Build history of the part. All positions in model axes, mm. Round coordinates to 2 decimals unless told otherwise and drop trailing zeros. Write each loop counter-clockwise with the first axis right and the second up, starting at its lowest first coordinate (ties: lowest second). Pieces come first, ordered by that corner, then holes. Notation, with made-up numbers: (76.5, -25.75) -> (132.5, -25.75) arc R22 cw to (132.5, -12.75) -> close; hole circle Ø1 at (77.25, 55). An arc over 180 degrees is marked (long way). Answer in a Markdown table with one row per item.
```python
from build123d import *

# Parameters (mm, degrees)
SZKIC2_R                         = 5
DODANIE_WYCI_GNI_CIE1_DEPTH      = 175
DODANIE_WYCI_GNI_CIE2_DEPTH      = 15
DODANIE_WYCI_GNI_CIE2_DEPTH_BACK = 15
SZKIC3_R                         = 1
ZAOKR_GLENIE1_R                  = 5


with BuildPart() as part:
    # Szkic2 → Dodanie-wyci_gni_cie1 (new body)
    with BuildSketch(Plane(origin=(0, 0, 0), x_dir=(1, 0, 0), z_dir=(0, 1, 0))):
        with Locations(Location((0, 0, 0), (0, 0, 270))):
            Circle(SZKIC2_R)
    extrude(amount=DODANIE_WYCI_GNI_CIE1_DEPTH)

    # Szkic3 → Dodanie-wyci_gni_cie2 (add, two sides: drawn at the far end of the back side and taken through both)
    with BuildSketch(Plane.XY.offset(-DODANIE_WYCI_GNI_CIE2_DEPTH_BACK)):
        with Locations((0, 95)):
            Circle(SZKIC3_R)
    extrude(amount=DODANIE_WYCI_GNI_CIE2_DEPTH + DODANIE_WYCI_GNI_CIE2_DEPTH_BACK)

    # Zaokr_glenie1
    zaokr_glenie1_edges = [part.edges().sort_by_distance(p)[0] for p in [
        (0, 0, -5),
    ]]
    fillet(zaokr_glenie1_edges, radius=ZAOKR_GLENIE1_R)


solid = part.part
```
Q1. Saw through at B-B on x = -3. Write the cut outline in (y, z).
A:
| item | result |
|---|---|
| outline | (5, -4) -> (175, -4) -> (175, 4) -> (5, 4) arc R4 ccw to start |
Q2. Wall check: line 1 (Y direction, x = -0.25, z = 9.5); line 2 (X direction, y = 103.5, z = 1); line 3 (Z direction, x = 0, y = 117.5). Give the ranges that are in metal, low to high. Write a range as [from, to].
A:
| item | result |
|---|---|
| line 1 | [94.03, 95.97] |
| line 2 | [-4.9, 4.9] |
| line 3 | [-5, 5] |
Q3. Saw through at A-A on y = 138. Write the cut outline in (x, z), plus the area to 3 significant figures.
A:
| item | result |
|---|---|
| outline | circle Ø10 at (0, 0) |
| area | 78.5 mm² |
Q4. Saw through at D-D on x = 3.5. Write the cut outline in (y, z).
A:
| item | result |
|---|---|
| outline | (5, -3.57) -> (175, -3.57) -> (175, 3.57) -> (5, 3.57) arc R3.57 ccw to start |
Q5. Saw through at C-C on z = -8.5. Write the cut outline in (x, y), plus the area to 3 significant figures.
A:
| item | result |
|---|---|
| outline | circle Ø2 at (0, 95) |
| area | 3.14 mm² |
Q6. Drop flat-ended pins along their axis: P1, Ø2, axis at x = -1, z = 11, coming from the -Y side; P2, Ø1, axis at x = 3, y = 85.5, coming from the +Z side; P3, Ø6, axis at y = 88.5, z = 4.5, coming from the -X side. Give the stop position or say it passes through.
A:
| item | result |
|---|---|
| P1 | y = 94 |
| P2 | z = 4.33 |
| P3 | x = -4.77 |
